Autodesk Inventor part; units mm, degrees
ref_plane "YZ Plane" through (0, 0, 0) normal (1, 0, 0) x (0, 1, 0)
ref_plane "XZ Plane" through (0, 0, 0) normal (0, 1, 0) x (-1, 0, 0)
ref_plane "XY Plane" through (0, 0, 0) normal (0, 0, 1) x (1, 0, 0)
sketch "Náčrt1" plane through (0, 0, 0) normal (0, 1, 0) x (-1, 0, 0)
  circle A0 centre (0, 0) radius 16.5
  circle A1 centre (0, 0) radius 13.5
  dimension "d0" = 33
  dimension "d1" = 27
extrude "Vysunutí1" add sketch "Náčrt1" along normal mid plane 25 contours A1
sketch "Náčrt4" plane through (0, 0, 0) normal (1, 0, 0) x (0, 1, 0)
  line L0 (-12.5, 13.5) -> (-12.5, -13.5)
  point P0 (0, 0)
  point P1 (-8.5, 0)
  dimension "d16" = 4
hole "Díra2" at (0, -8.5, 0) direction (1, 0, 0) diameter 3 end through all
thread "Závit1"
extrude "Vysunutí2" add sketch "Náčrt1" along normal mid plane 22
sketch "Náčrt2" plane through (0, 12.5, 0) normal (0, 1, 0) x (1, 0, 0)
  circle A0 centre (0, 0) radius 9
  dimension "d6" = 18
extrude "Vysunutí3" cut sketch "Náčrt2" against normal blind 14.5
sketch "Náčrt3" plane through (0, -12.5, 0) normal (0, -1, 0) x (1, 0, 0)
  circle A0 centre (0, 0) radius 13.5
hole "Díra1" at (0, -12.5, 0) direction (0, 1, 0) diameter 3 end through all
sketch "Náčrt5" plane through (0, -11, 0) normal (0, -1, 0) x (1, 0, 0)
  circle A0 centre (0, 0) radius 16.5
  circle A1 centre (0, 0) radius 12
  dimension "d26" = 24
extrude "Vysunutí4" cut sketch "Náčrt5" against normal up to surface (22 mm away)
properties part number "JSUMO_Wheel_33x25mm_NoSilicon"
Geometry: final body of the model. Coordinates: model frame, mm. A direction names the side the tool comes from. Give positions to 0.01 mm unless a question says otherwise; leave off trailing zeros. Loops run counter-clockwise (first coordinate to the right, second up) from the corner with the lowest first, then second, coordinate; pieces in that order, holes last. Notation, with made-up numbers: (46, 13.25) -> (62, 13.25) arc R26 cw to (62, 31.25) -> close; hole circle Ø3 at (79, -35.5). An arc over 180 degrees is marked (long way). Return JSON: item names as keys, results as strings.
Item 1: Section A-A, the plane z = 0. Output: boundary loops of the cut face in (x, y).
Filled in:
{"outline": "(-13.5, -12.5) -> (-1.5, -12.5) -> (-1.5, -2) -> (-9, -2) -> (-9, 12.5) -> (-13.5, 12.5) -> (-13.5, 11) -> (-12, 11) -> (-12, -11) -> (-13.5, -11) -> close; (1.5, -12.5) -> (13.5, -12.5) -> (13.5, -11) -> (12, -11) -> (12, -10) -> (1.5, -10) -> close; (1.5, -7) -> (12, -7) -> (12, 11) -> (13.5, 11) -> (13.5, 12.5) -> (9, 12.5) -> (9, -2) -> (1.5, -2) -> close"}
Item 2: Section B-B, the plane y = -6. Output: boundary loops of the cut face in (x, z), plus the area to 3 significant figures.
Filled in:
{"outline": "circle Ø24 at (0, 0); hole circle Ø3 at (0, 0)", "area": "445 mm^2"}
Item 3: Section D-D, the plane y = 8.5. Output: boundary loops of the cut face in (x, z).
Filled in:
{"outline": "circle Ø24 at (0, 0); hole circle Ø18 at (0, 0)"}
Item 4: Section C-C, the plane z = 10.5. Output: boundary loops of the cut face in (x, y), plus the area to 3 significant figures.
Filled in:
{"outline": "(-8.49, -12.5) -> (8.49, -12.5) -> (8.49, -11) -> (5.81, -11) -> (5.81, 11) -> (8.49, 11) -> (8.49, 12.5) -> (-8.49, 12.5) -> (-8.49, 11) -> (-5.81, 11) -> (-5.81, -11) -> (-8.49, -11) -> close", "area": "307 mm^2"}
Item 5: Mould query, pull axis X, two halves, no side actions, for faces 1 (the cylindrical face through (2.93, 11.74, 13.18)), 2 (the cylindrical face through (-1.487, -7.176, 0.195)), 3 (the flat face through (-3, -12.5, 0)). Classes: released by +X, released by -X, zero draft, split by the parting line, or undercut.
Filled in:
{"face 1": "split by the parting line", "face 2": "undercut", "face 3": "zero draft"}
Item 6: Pin query (flat end, axial travel): P1, Ø5, axis at y = -9, z = 8.5, coming from the -X side; P2, Ø3.5, axis at x = 0, z = 0, coming from the +Y side; P3, Ø14.5, axis at x = -3.5, z = -3, coming from the +Y side; P4, Ø6, axis at y = 6.5, z = 9.5, coming from the +X side. Return the tip coordinate at first contact, or that it passes through.
Filled in:
{"P1": "x = -11.54", "P2": "y = -2", "P3": "y = 12.5", "P4": "x = 10.09"}
Item 7: Access query for faces 4 (the flat face through (-9, 12.5, -3)), 5 (the cylindrical face through (-11.99, -0.15, 0.53)), 6 (the cylindrical face through (-1.172, 5.352, -8.923)), 7 (the cylindrical face through (6.084, -7.925, 1.386)). Directions: +Z, -Z, +X, -X, +Y, -Y. A direction counts if a zero-diameter tool reaches every point of the face in a straight line with its end or side. Return the directions, or none.
Filled in:
{"face 4": "+Z, -Z, +X, -X, +Y", "face 5": "none", "face 6": "+Y", "face 7": "+X"}
Item 8: Line query: line 1 (Z direction, x = 0, y = 8); line 2 (Z direction, x = 0, y = -5.75); line 3 (Y direction, x = 8.5, z = 0). Output: solid intervals per line, ascending.
Filled in:
{"line 1": "-12 to -9, 9 to 12", "line 2": "-12 to -1.5, 1.5 to 12", "line 3": "-12.5 to -10, -7 to -2"}
